Input: part model. Units: mm. Frame: model coordinates. Round coordinates to 2 decimals unless told otherwise and drop trailing zeros. Write each loop counter-clockwise with the first axis right and the second up, starting at its lowest first coordinate (ties: lowest second). Pieces come first, ordered by that corner, then holes. Notation, with made-up numbers: (75.25, -7.75) -> (96.25, -7.75) arc R24 ccw to (96.25, 4.25) -> close; hole circle Ø4 at (-8, 34.5). An arc over 180 degrees is marked (long way). Use CSV: the item, a comma, the result in double quotes.
```python
from build123d import *

# Parameters (mm, degrees)
F0_R     = 6.35
F1_DEPTH = 1


with BuildPart() as f1:
    # F0 (on Top) → F1 (new body)
    with BuildSketch(Plane.XY):
        with BuildLine():
            ThreePointArc((-3.9687500424, -6.8740766181), (-7.6670362525, -2.0543761469), (-6.8740766425, 3.96875))
            Line((-6.8740766425, 3.96875), (-14.8115766425, -9.7794032851))
            ThreePointArc((-14.8115766425, -9.7794032851), (-9.9918761941, -6.0811170452), (-3.9687500424, -6.8740766181))
        make_face()
        with BuildLine():
            ThreePointArc((0, -13.7481532851), (-1.0634233697, -9.7794032639), (-3.9687500424, -6.8740766181))
            ThreePointArc((-3.9687500424, -6.8740766181), (-9.9918761941, -6.0811170452), (-14.8115766425, -9.7794032851))
            ThreePointArc((-14.8115766425, -9.7794032851), (-14.8115766425, -17.7169032851), (-7.9375, -21.6856532851))
            ThreePointArc((-7.9375, -21.6856532851), (-2.3248399243, -19.3608133607), (0, -13.7481532851))
        make_face()
        with Locations((-7.9375, -13.7481532851)):
            Circle(F0_R, mode=Mode.SUBTRACT)
        with BuildLine():
            ThreePointArc((7.9375, -21.6856532851), (2.3248399243, -19.3608133607), (0, -13.7481532851))
            ThreePointArc((0, -13.7481532851), (-2.3248399243, -19.3608133607), (-7.9375, -21.6856532851))
            Line((-7.9375, -21.6856532851), (7.9375, -21.6856532851))
        make_face()
        with BuildLine():
            ThreePointArc((14.8115766425, -9.7794032851), (9.9918761512, -6.0811170337), (3.9687499653, -6.8740766625))
            ThreePointArc((3.9687499653, -6.8740766625), (1.0634233475, -9.7794033024), (0, -13.7481532851))
            ThreePointArc((0, -13.7481532851), (2.3248399243, -19.3608133607), (7.9375, -21.6856532851))
            ThreePointArc((7.9375, -21.6856532851), (13.5501600757, -19.3608133607), (15.875, -13.7481532851))
            ThreePointArc((15.875, -13.7481532851), (15.6045362462, -11.6937771146), (14.8115766425, -9.7794032851))
        make_face()
        with Locations((7.9375, -13.7481532851)):
            Circle(F0_R, mode=Mode.SUBTRACT)
        with BuildLine():
            ThreePointArc((6.8740766425, 3.96875), (7.6670362462, 2.0543761705), (7.9375, 0))
            ThreePointArc((7.9375, 0), (6.8740766325, -3.9687500173), (3.9687499653, -6.8740766625))
            ThreePointArc((3.9687499653, -6.8740766625), (9.9918761512, -6.0811170337), (14.8115766425, -9.7794032851))
            Line((14.8115766425, -9.7794032851), (6.8740766425, 3.96875))
        make_face()
        with BuildLine():
            ThreePointArc((0, -13.7481532851), (1.0634233475, -9.7794033024), (3.9687499653, -6.8740766625))
            ThreePointArc((3.9687499653, -6.8740766625), (-4.45e-08, -7.9375), (-3.9687500424, -6.8740766181))
            ThreePointArc((-3.9687500424, -6.8740766181), (-1.0634233697, -9.7794032639), (0, -13.7481532851))
        make_face()
        with BuildLine():
            ThreePointArc((3.9687499653, -6.8740766625), (6.8740766325, -3.9687500173), (7.9375, 0))
            ThreePointArc((7.9375, 0), (7.6670362462, 2.0543761705), (6.8740766425, 3.96875))
            ThreePointArc((6.8740766425, 3.96875), (0, 7.9375), (-6.8740766425, 3.96875))
            ThreePointArc((-6.8740766425, 3.96875), (-7.6670362525, -2.0543761469), (-3.9687500424, -6.8740766181))
            ThreePointArc((-3.9687500424, -6.8740766181), (-4.45e-08, -7.9375), (3.9687499653, -6.8740766625))
        make_face()
        Circle(F0_R, mode=Mode.SUBTRACT)
    extrude(amount=F1_DEPTH)


solid = f1.part
```
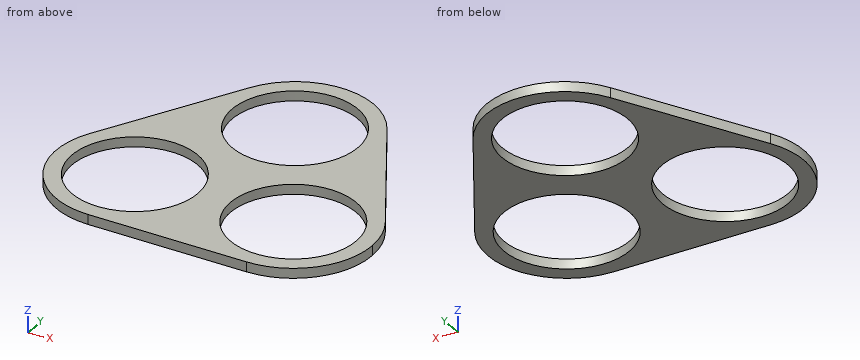
Item 1: Section query C-C on z = 0.35. Give the number of separate pieces and of enclosed holes in the cut face, plus the area to 3 significant figures.
Worked answers:
separate pieces,"1"
enclosed holes,"3"
area,"305 mm²"
Item 2: Section query B-B on y = -13. Return the cut outline in (x, z), plus the area to 3 significant figures.
Worked answers:
outline,"(-15.84, 0) -> (-14.24, 0) -> (-14.24, 1) -> (-15.84, 1) -> close; (-1.63, 0) -> (1.63, 0) -> (1.63, 1) -> (-1.63, 1) -> close; (14.24, 0) -> (15.84, 0) -> (15.84, 1) -> (14.24, 1) -> close"
area,"6.46 mm²"
Item 3: Section query D-D on y = 5.5. Return the cut outline in (x, z), plus the area to 3 significant figures.
Worked answers:
outline,"(-5.72, 0) -> (-3.17, 0) -> (-3.17, 1) -> (-5.72, 1) -> close; (3.17, 0) -> (5.72, 0) -> (5.72, 1) -> (3.17, 1) -> close"
area,"5.10 mm²"
Item 4: Section query A-A on x = 0. Return the cut outline in (y, z), plus the area to 3 significant figures.
Worked answers:
outline,"(-21.69, 0) -> (-6.35, 0) -> (-6.35, 1) -> (-21.69, 1) -> close; (6.35, 0) -> (7.94, 0) -> (7.94, 1) -> (6.35, 1) -> close"
area,"16.9 mm²"
Item 5: Line query: line 1 (X direction, y = -18.25, z = 0.8); line 2 (Y direction, x = -5, z = 0.2); line 3 (X direction, y = -9.5, z = 0.15). Output: solid intervals per line, ascending.
Worked answers:
line 1,"x = -14.47 to -12.42, -3.46 to 3.46, 12.42 to 14.47"
line 2,"y = -21.69 to -19.38, -8.12 to -3.91, 3.91 to 6.16"
line 3,"x = -14.65 to -12.66, -3.22 to 3.22, 12.66 to 14.65"
